```python
from build123d import *

# Parameters (mm, degrees)
BASE_EXTRUDE_DEPTH   = 30
CUT_EXTRUDE1_DEPTH   = 6
FILLET1_R            = 6
FILLET1_OF_MIRROR1_R = 6
MIRROR2_START        = -8
MIRROR2_DEPTH        = 6
MIRROR2_START_2      = 2
MIRROR2_2_DEPTH      = 6
SKETCH5_W            = 16
SKETCH5_H            = 75
CUT_EXTRUDE3_DEPTH   = 1.5


# Read off the part's stored shape, not the designer's step: Mirror2
with BuildPart() as part:
    # Sketch1 → Base-Extrude (new body)
    with BuildSketch(Plane(origin=(0, 0, 0), x_dir=(1, 0, 0), z_dir=(0, 1, 0))):
        with BuildLine():
            Line((8, 37.5), (2.993373056, 112.699293126))
            ThreePointArc((2.993373056, 112.699293126), (0, 115.5), (-2.993373056, 112.699293126))
            Line((-2.993373056, 112.699293126), (-8, 37.5))
            Line((-8, 37.5), (-8, -37.5))
            Line((-8, -37.5), (-2.993373056, -112.699293126))
            ThreePointArc((-2.993373056, -112.699293126), (0, -115.5), (2.993373056, -112.699293126))
            Line((2.993373056, -112.699293126), (8, -37.5))
            Line((8, -37.5), (8, 37.5))
        make_face()
    extrude(amount=BASE_EXTRUDE_DEPTH)

    # Sketch2 → Cut-Extrude1 (cut)
    with BuildSketch(Plane(origin=(8, 0, 0), x_dir=(0, 0, -1), z_dir=(1, 0, 0))):
        with BuildLine():
            Line((-37.5, 5), (-95.5, 5))
            ThreePointArc((-95.5, 5), (-105.5, 15), (-95.5, 25))
            Line((-95.5, 25), (-37.5, 25))
            Line((-37.5, 25), (-37.5, 5))
        make_face()
    cut_extrude1 = extrude(amount=-CUT_EXTRUDE1_DEPTH, mode=Mode.SUBTRACT)

    # Fillet1
    fillet1_edges = [part.edges().sort_by_distance(p)[0] for p in [
        (5, 25, 37.5),
        (5, 5, 37.5),
    ]]
    fillet(fillet1_edges, radius=FILLET1_R)

    # Mirror1: Cut-Extrude1 across plane
    add(cut_extrude1.mirror(Plane(origin=(0, 0, 0), x_dir=(0, 0, 1), z_dir=(1, 0, 0))), mode=Mode.SUBTRACT)

    # Fillet1 of Mirror1
    fillet1_of_mirror1_edges = [part.edges().sort_by_distance(p)[0] for p in [
        (-5, 25, 37.5),
        (-5, 5, 37.5),
    ]]
    fillet(fillet1_of_mirror1_edges, radius=FILLET1_OF_MIRROR1_R)

    # Mirror2 outline → Mirror2 (cut)
    with BuildSketch(Plane.YZ.offset(MIRROR2_START)):
        with BuildLine():
            Line((5, -43.5), (5, -95.5))
            ThreePointArc((5, -95.5), (15, -105.5), (25, -95.5))
            Line((25, -95.5), (25, -43.5))
            ThreePointArc((25, -43.5), (23.242640687, -39.257359313), (19, -37.5))
            Line((19, -37.5), (11, -37.5))
            ThreePointArc((11, -37.5), (6.757359313, -39.257359313), (5, -43.5))
        make_face()
    extrude(amount=MIRROR2_DEPTH, mode=Mode.SUBTRACT)

    # Mirror2 2 outline → Mirror2 2 (cut)
    with BuildSketch(Plane.YZ.offset(MIRROR2_START_2)):
        with BuildLine():
            Line((5, -43.5), (5, -95.5))
            ThreePointArc((5, -95.5), (15, -105.5), (25, -95.5))
            Line((25, -95.5), (25, -43.5))
            ThreePointArc((25, -43.5), (23.242640687, -39.257359313), (19, -37.5))
            Line((19, -37.5), (11, -37.5))
            ThreePointArc((11, -37.5), (6.757359313, -39.257359313), (5, -43.5))
        make_face()
    extrude(amount=MIRROR2_2_DEPTH, mode=Mode.SUBTRACT)

    # Sketch5 → Cut-Extrude3 (cut)
    with BuildSketch(Plane(origin=(0, 30, 0), x_dir=(-1, 0, 0), z_dir=(0, 1, 0))):
        Rectangle(SKETCH5_W, SKETCH5_H)
    extrude(amount=-CUT_EXTRUDE3_DEPTH, mode=Mode.SUBTRACT)


solid = part.part
```
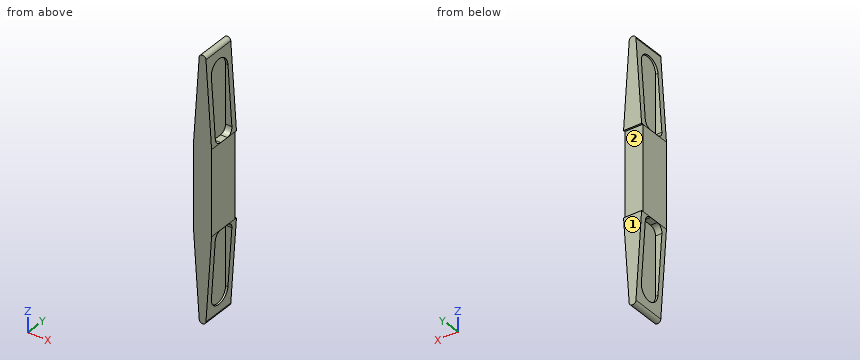
The listing builds one solid part. Answer for the finished solid, in the listing's coordinates (mm). Face numbers are marked on the shaded views. Coordinates: 2 decimals unless noted, no trailing zeros. Write each loop counter-clockwise with the first axis right and the second up, starting at its lowest first coordinate (ties: lowest second). Pieces come first, ordered by that corner, then holes. Notation, with made-up numbers: M 63.5,22.25 L 84.5,22.25 A13 ccw 84.5,34.25 Z; hole C -25.75,-15.75 d3. An arc over 180 degrees is marked long. Use a Markdown table: item, result. Add a question column.
1. Section B-B (z = -98) is taken. Give the vertices of the cut face in (x, y).
2. Straight lines are drawn through the part: line 1 along Y through (x, z) = (5, -68.5); line 2 along X through (y, z) = (24, 71); line 3 along Z through (x, y) = (-2.5, 24). For each, find the intervals that lie inside material, in ascending order. Write a range as [from, to].
3. Section D-D (z = 5) is taken. Give the vertices of the cut face in (x, y).
4. For a pull along Z with two mould halves and no side action, classify the marked faces 1 and 2 as +Z half, -Z half, draft (parallel to the pull), parting line (faces both ways), or undercut.
5. Given P1, Ø16, axis at y = 11.5, z = -62, coming from the -X side; P2, Ø2, axis at x = 6.5, y = 15, coming from the -Z side; P3, Ø5, axis at x = 3, z = 5, coming from the +Y side, each flat-ended and moving along its own axis, determine where each tip first touches the part or whether it passes through.
6. Section C-C (z = -40.5) is taken. Give the vertices of the cut face in (x, y), plus the area to 3 significant figures.
7. Section A-A (x = 0) is taken. Give the vertices of the cut face in (y, z).
Data:
| question | item | result |
|---|---|---|
| 1 | outline | M -3.97,0 L 3.97,0 L 3.97,5.32 L 2,5.32 L 2,24.68 L 3.97,24.68 L 3.97,30 L -3.97,30 L -3.97,24.68 L -2,24.68 L -2,5.32 L -3.97,5.32 Z |
| 2 | line 1 | y = [0, 5], [25, 30] |
| 2 | line 2 | x = [-2, 2] |
| 2 | line 3 | z = [-114.16, -99.86], [-40.18, 40.18], [99.86, 114.16] |
| 3 | outline | M -8,0 L 8,0 L 8,28.5 L -8,28.5 Z |
| 4 | face 1 | draft |
| 4 | face 2 | undercut |
| 5 | P1 | stops at x = -6.68 |
| 5 | P2 | stops at z = -37.5 |
| 5 | P3 | stops at y = 28.5 |
| 6 | outline | M -7.8,0 L 7.8,0 L 7.8,5.8 L 2,5.8 L 2,24.2 L 7.8,24.2 L 7.8,30 L -7.8,30 L -7.8,24.2 L -2,24.2 L -2,5.8 L -7.8,5.8 Z |
| 6 | area | 255 mm2 |
| 7 | outline | M 0,-115.5 L 30,-115.5 L 30,-37.5 L 28.5,-37.5 L 28.5,37.5 L 30,37.5 L 30,115.5 L 0,115.5 Z |
